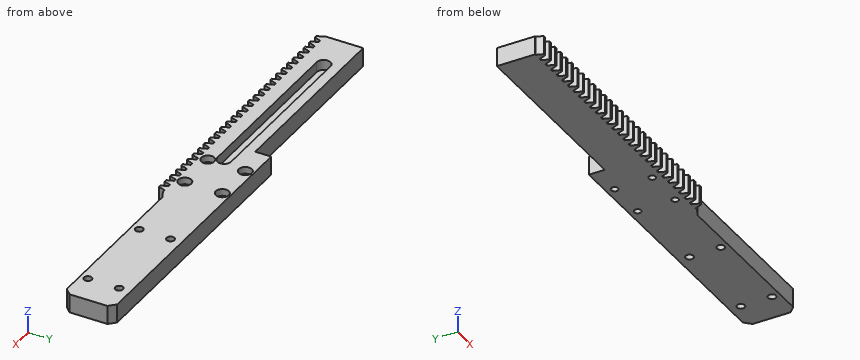
```python
from build123d import *

# Parameters (mm, degrees)
MODULE_START                                   = 40.4
MODULE_1_RACK_WITH_VERTICAL_CARRIER_TAIL_DEPTH = 6
MGN7H_START                                    = 40.4
MGN7H_CARRIAGE_FIXING_PAD_PROFILE_W            = 33
MGN7H_CARRIAGE_FIXING_PAD_PROFILE_H            = 6.1
MGN7H_CARRIAGE_FIXING_PAD_DEPTH                = 6
FULL_START                                     = 43.1
FULL_STROKE_LIMIT_SLOT_56_55_MM_DEPTH          = 3.4
RADAR_START                                    = 40.3
RADAR_SEAT_FOUR_M3_PILOTS_29_X_10_MM_PRO_R     = 1.25
RADAR_SEAT_FOUR_M3_PILOTS_29_X_10_MM_DEPTH     = 6.2
MGN7H_START_2                                  = 40.3
MGN7H_FOUR_M2_CLEARANCES_13_X_12_MM_PROF_R     = 1.1
MGN7H_FOUR_M2_CLEARANCES_13_X_12_MM_DEPTH      = 6.2
MGN7H_START_3                                  = 44.2
MGN7H_M2_HEAD_POCKETS_PROFILE_R                = 2.1
MGN7H_M2_HEAD_POCKETS_DEPTH                    = 2.3


with BuildPart() as part:
    # Module 1 rack with vertical carrier  2 → Module 1 rack with vertical carrier tail (new body)
    with BuildSketch(Plane.XY.offset(MODULE_START)):
        Polygon((-69, 10.26), (-68.713242711, 10.26), (-67.908868493, 8.05), (-67.179615611, 8.05), (-66.375241394, 10.26), (-65.571650057, 10.26), (-64.767275839, 8.05), (-64.038022958, 8.05), (-63.23364874, 10.26), (-62.430057404, 10.26), (-61.625683186, 8.05), (-60.896430304, 8.05), (-60.092056086, 10.26), (-59.28846475, 10.26), (-58.484090532, 8.05), (-57.754837651, 8.05), (-56.950463433, 10.26), (-56.146872096, 10.26), (-55.342497879, 8.05), (-54.613244997, 8.05), (-53.808870779, 10.26), (-53.005279443, 10.26), (-52.200905225, 8.05), (-51.471652343, 8.05), (-50.667278126, 10.26), (-49.863686789, 10.26), (-49.059312572, 8.05), (-48.33005969, 8.05), (-47.525685472, 10.26), (-46.722094136, 10.26), (-45.917719918, 8.05), (-45.188467036, 8.05), (-44.384092819, 10.26), (-43.580501482, 10.26), (-42.776127264, 8.05), (-42.046874383, 8.05), (-41.242500165, 10.26), (-40.438908828, 10.26), (-39.634534611, 8.05), (-38.905281729, 8.05), (-38.100907511, 10.26), (-37.297316175, 10.26), (-36.492941957, 8.05), (-35.763689075, 8.05), (-34.959314858, 10.26), (-34.155723521, 10.26), (-33.351349304, 8.05), (-32.622096422, 8.05), (-31.817722204, 10.26), (-31.014130868, 10.26), (-30.20975665, 8.05), (-29.480503768, 8.05), (-28.676129551, 10.26), (-27.872538214, 10.26), (-27.068163996, 8.05), (-26.338911115, 8.05), (-25.534536897, 10.26), (-24.730945561, 10.26), (-23.926571343, 8.05), (-23.197318461, 8.05), (-22.392944243, 10.26), (-21.589352907, 10.26), (-20.784978689, 8.05), (-20.055725808, 8.05), (-19.25135159, 10.26), (-18.447760253, 10.26), (-17.643386036, 8.05), (-16.914133154, 8.05), (-16.109758936, 10.26), (-15.3061676, 10.26), (-14.501793382, 8.05), (-13.7725405, 8.05), (-12.968166283, 10.26), (-12.164574946, 10.26), (-11.360200728, 8.05), (-10.630947847, 8.05), (-9.826573629, 10.26), (-9.022982293, 10.26), (-8.218608075, 8.05), (-7.489355193, 8.05), (-6.684980975, 10.26), (-5.881389639, 10.26), (-5.077015421, 8.05), (-4.34776254, 8.05), (-3.543388322, 10.26), (-2.739796985, 10.26), (-1.935422768, 8.05), (-1.206169886, 8.05), (-0.401795668, 10.26), (0.401795668, 10.26), (1.206169886, 8.05), (1.935422768, 8.05), (2.739796985, 10.26), (3.543388322, 10.26), (4.34776254, 8.05), (5.077015421, 8.05), (5.881389639, 10.26), (6.684980975, 10.26), (7.489355193, 8.05), (8.218608075, 8.05), (9.022982293, 10.26), (9.826573629, 10.26), (10.630947847, 8.05), (11.360200728, 8.05), (12.164574946, 10.26), (12.968166283, 10.26), (13.7725405, 8.05), (14.501793382, 8.05), (15.3061676, 10.26), (16.109758936, 10.26), (16.914133154, 8.05), (17.643386036, 8.05), (18.447760253, 10.26), (19.25135159, 10.26), (20.055725808, 8.05), (20.784978689, 8.05), (21.589352907, 10.26), (22.5, 10.26), (25, 11.5), (79, 11.5), (81, 13.5), (81, 25.6), (79, 27.6), (22.5, 27.6), (22.5, 22.5), (-69, 22.5), align=None)
    extrude(amount=MODULE_1_RACK_WITH_VERTICAL_CARRIER_TAIL_DEPTH)

    # MGN7H carriage fixing pad profile → MGN7H carriage fixing pad (add)
    with BuildSketch(Plane.XY.offset(MGN7H_START)):
        with Locations((8.5, 24.55)):
            Rectangle(MGN7H_CARRIAGE_FIXING_PAD_PROFILE_W, MGN7H_CARRIAGE_FIXING_PAD_PROFILE_H)
    extrude(amount=MGN7H_CARRIAGE_FIXING_PAD_DEPTH)

    # Full stroke limit slot 56.55 mm profile → Full stroke limit slot 56.55 mm (cut)
    with BuildSketch(Plane.XY.offset(FULL_START)):
        with BuildLine():
            Line((-56.348667765, 14.8), (-0.2, 14.8))
            ThreePointArc((-0.2, 14.8), (2, 17), (-0.2, 19.2))
            Line((-0.2, 19.2), (-56.348667765, 19.2))
            ThreePointArc((-56.348667765, 19.2), (-58.548667765, 17), (-56.348667765, 14.8))
        make_face()
    extrude(amount=FULL_STROKE_LIMIT_SLOT_56_55_MM_DEPTH, mode=Mode.SUBTRACT)

    # Radar seat four M3 pilots 29 x 10 mm profile → Radar seat four M3 pilots 29 x 10 mm (cut)
    with BuildSketch(Plane.XY.offset(RADAR_START)):
        with Locations(Location((42.5, 14, 0), (0, 0, 180))):
            Circle(RADAR_SEAT_FOUR_M3_PILOTS_29_X_10_MM_PRO_R)
        with Locations(Location((42.5, 24, 0), (0, 0, 180))):
            Circle(RADAR_SEAT_FOUR_M3_PILOTS_29_X_10_MM_PRO_R)
        with Locations(Location((71.5, 14, 0), (0, 0, 180))):
            Circle(RADAR_SEAT_FOUR_M3_PILOTS_29_X_10_MM_PRO_R)
        with Locations(Location((71.5, 24, 0), (0, 0, 180))):
            Circle(RADAR_SEAT_FOUR_M3_PILOTS_29_X_10_MM_PRO_R)
    extrude(amount=RADAR_SEAT_FOUR_M3_PILOTS_29_X_10_MM_DEPTH, mode=Mode.SUBTRACT)

    # MGN7H four M2 clearances 13 x 12 mm profile → MGN7H four M2 clearances 13 x 12 mm (cut)
    with BuildSketch(Plane.XY.offset(MGN7H_START_2)):
        with Locations(Location((2, 13, 0), (0, 0, 180))):
            Circle(MGN7H_FOUR_M2_CLEARANCES_13_X_12_MM_PROF_R)
        with Locations(Location((2, 25, 0), (0, 0, 180))):
            Circle(MGN7H_FOUR_M2_CLEARANCES_13_X_12_MM_PROF_R)
        with Locations(Location((15, 13, 0), (0, 0, 180))):
            Circle(MGN7H_FOUR_M2_CLEARANCES_13_X_12_MM_PROF_R)
        with Locations(Location((15, 25, 0), (0, 0, 180))):
            Circle(MGN7H_FOUR_M2_CLEARANCES_13_X_12_MM_PROF_R)
    extrude(amount=MGN7H_FOUR_M2_CLEARANCES_13_X_12_MM_DEPTH, mode=Mode.SUBTRACT)

    # MGN7H M2 head pockets profile → MGN7H M2 head pockets (cut)
    with BuildSketch(Plane.XY.offset(MGN7H_START_3)):
        with Locations((2, 13)):
            Circle(MGN7H_M2_HEAD_POCKETS_PROFILE_R)
        with Locations((2, 25)):
            Circle(MGN7H_M2_HEAD_POCKETS_PROFILE_R)
        with Locations((15, 13)):
            Circle(MGN7H_M2_HEAD_POCKETS_PROFILE_R)
        with Locations((15, 25)):
            Circle(MGN7H_M2_HEAD_POCKETS_PROFILE_R)
    extrude(amount=MGN7H_M2_HEAD_POCKETS_DEPTH, mode=Mode.SUBTRACT)


solid = part.part
```
Verification items for the finished model (mm, model axes). Coordinates: 2 decimals unless noted, no trailing zeros. Write each loop counter-clockwise with the first axis right and the second up, starting at its lowest first coordinate (ties: lowest second). Pieces come first, ordered by that corner, then holes. Notation, with made-up numbers: (-10.5, -27.5) - (43.5, -27.5) arc R17 ccw to (43.5, -15.5) - close; hole circle Ø7 at (79.25, 48.25). An arc over 180 degrees is marked (long way). One line per question, with ' | ' between items. Start each with the question number.
1. Section check A-A (x = 42.5). Enter the section's corners in (y, z).
2. Section check B-B (y = 17). Enter the section's corners in (x, z).
3. Gauge pin test, flat ends, axial feed: P1, Ø1.3, axis at x = 2, y = 12, coming from the +Z side; P2, Ø0.6, axis at x = 0, z = 42.5, coming from the -Y side; P3, Ø3, axis at y = 10.5, z = 43.5, coming from the +X side. Record the tip position at first contact, or that the pin passes through.
4. Section check C-C (z = 41.45). Count the separate pieces of the cut face and the enclosed holes in it, plus the area to 3 significant figures.
5. Material ranges on line 1 along Y through (x, z) = (-53.5, 45.15); line 2 along X through (y, z) = (23.25, 41.1); line 3 along Z through (x, y) = (-14, 15.25), recorded low to high.
Computed values:
1) outline: (11.5, 40.4) - (12.75, 40.4) - (12.75, 46.4) - (11.5, 46.4) - close; (15.25, 40.4) - (22.75, 40.4) - (22.75, 46.4) - (15.25, 46.4) - close; (25.25, 40.4) - (27.6, 40.4) - (27.6, 46.4) - (25.25, 46.4) - close
2) outline: (-69, 40.4) - (81, 40.4) - (81, 46.4) - (2, 46.4) - (2, 43.1) - (-58.55, 43.1) - (-58.55, 46.4) - (-69, 46.4) - close
3) P1: z = 44.2 | P2: y = 10.26 | P3: x = 79.5
4) separate pieces: 1 | enclosed holes: 8 | area: 2,280 mm²
5) line 1: 10.26 to 14.8, 19.2 to 22.5 | line 2: -8 to 41.5, 43.5 to 70.5, 72.5 to 81 | line 3: 40.4 to 43.1
